from build123d import *

# Parameters (mm, degrees)
F1_DEPTH      = 125
F1_DEPTH_BACK = 125
F6_DEPTH      = 5.001
F7_DEPTH      = 30.001
F8_DEPTH      = 2
F9_DEPTH      = 2
F10_DEPTH     = 2
F11_DEPTH     = 2


with BuildPart() as f1:
    # F0 (on Front) → F1 (new body, two sides)
    with BuildSketch(Plane.XZ) as f1_sk:
        Polygon((15, -20), (15, 20), (-15, 20), (-15, -20), (-10, -20), (-10, 15), (10, 15), (10, -20), align=None)
    extrude(amount=F1_DEPTH)
    extrude(f1_sk.sketch, amount=-F1_DEPTH_BACK)

    # F4 (on face) → F6 (cut, through all)
    with BuildSketch(Plane.YZ.offset(-10)):
        with BuildLine():
            Line((107.5, 2.5), (-107.5, 2.5))
            ThreePointArc((-107.5, 2.5), (-112.5, -2.5), (-107.5, -7.5))
            Line((-107.5, -7.5), (107.5, -7.5))
            ThreePointArc((107.5, -7.5), (112.5, -2.5), (107.5, 2.5))
        make_face()
    extrude(amount=-F6_DEPTH, mode=Mode.SUBTRACT)

    # F2 (on face) → F7 (cut, through all)
    with BuildSketch(Plane(origin=(-15, 0, 0), x_dir=(0, -1, 0), z_dir=(-1, 0, 0))):
        with BuildLine():
            Line((-107.5, -7.5), (107.5, -7.5))
            ThreePointArc((107.5, -7.5), (112.5, -2.5), (107.5, 2.5))
            Line((107.5, 2.5), (-107.5, 2.5))
            ThreePointArc((-107.5, 2.5), (-112.5, -2.5), (-107.5, -7.5))
        make_face()
    extrude(amount=-F7_DEPTH, mode=Mode.SUBTRACT)

    # F5 (on face) → F8 (cut)
    with BuildSketch(Plane(origin=(10, 0, 0), x_dir=(0, -1, 0), z_dir=(-1, 0, 0))):
        with BuildLine():
            Line((107.5, 8.75), (-107.5, 8.75))
            ThreePointArc((-107.5, 8.75), (-118.75, -2.5), (-107.5, -13.75))
            Line((-107.5, -13.75), (107.5, -13.75))
            ThreePointArc((107.5, -13.75), (118.75, -2.5), (107.5, 8.75))
        make_face()
        with BuildLine():
            ThreePointArc((-107.5, -7.5), (-112.5, -2.5), (-107.5, 2.5))
            Line((-107.5, 2.5), (107.5, 2.5))
            ThreePointArc((107.5, 2.5), (112.5, -2.5), (107.5, -7.5))
            Line((107.5, -7.5), (-107.5, -7.5))
        make_face(mode=Mode.SUBTRACT)
    extrude(amount=-F8_DEPTH, mode=Mode.SUBTRACT)

    # F4 (on face) → F9 (cut)
    with BuildSketch(Plane.YZ.offset(-10)):
        with BuildLine():
            Line((107.5, 8.75), (-107.5, 8.75))
            ThreePointArc((-107.5, 8.75), (-118.75, -2.5), (-107.5, -13.75))
            Line((-107.5, -13.75), (107.5, -13.75))
            ThreePointArc((107.5, -13.75), (118.75, -2.5), (107.5, 8.75))
        make_face()
        with BuildLine():
            ThreePointArc((-107.5, -7.5), (-112.5, -2.5), (-107.5, 2.5))
            Line((-107.5, 2.5), (107.5, 2.5))
            ThreePointArc((107.5, 2.5), (112.5, -2.5), (107.5, -7.5))
            Line((107.5, -7.5), (-107.5, -7.5))
        make_face(mode=Mode.SUBTRACT)
    extrude(amount=-F9_DEPTH, mode=Mode.SUBTRACT)

    # F3 (on face) → F10 (cut)
    with BuildSketch(Plane.YZ.offset(15)):
        with BuildLine():
            ThreePointArc((-107.5, 8.75), (-118.75, -2.5), (-107.5, -13.75))
            Line((-107.5, -13.75), (107.5, -13.75))
            ThreePointArc((107.5, -13.75), (118.75, -2.5), (107.5, 8.75))
            Line((107.5, 8.75), (-107.5, 8.75))
        make_face()
        with BuildLine():
            ThreePointArc((-107.5, -7.5), (-112.5, -2.5), (-107.5, 2.5))
            Line((-107.5, 2.5), (107.5, 2.5))
            ThreePointArc((107.5, 2.5), (112.5, -2.5), (107.5, -7.5))
            Line((107.5, -7.5), (-107.5, -7.5))
        make_face(mode=Mode.SUBTRACT)
    extrude(amount=-F10_DEPTH, mode=Mode.SUBTRACT)

    # F2 (on face) → F11 (cut)
    with BuildSketch(Plane(origin=(-15, 0, 0), x_dir=(0, -1, 0), z_dir=(-1, 0, 0))):
        with BuildLine():
            Line((-107.5, -13.75), (107.5, -13.75))
            ThreePointArc((107.5, -13.75), (118.75, -2.5), (107.5, 8.75))
            Line((107.5, 8.75), (-107.5, 8.75))
            ThreePointArc((-107.5, 8.75), (-118.75, -2.5), (-107.5, -13.75))
        make_face()
        with BuildLine():
            ThreePointArc((107.5, 2.5), (112.5, -2.5), (107.5, -7.5))
            Line((107.5, -7.5), (-107.5, -7.5))
            ThreePointArc((-107.5, -7.5), (-112.5, -2.5), (-107.5, 2.5))
            Line((-107.5, 2.5), (107.5, 2.5))
        make_face(mode=Mode.SUBTRACT)
    extrude(amount=-F11_DEPTH, mode=Mode.SUBTRACT)


solid = f1.part
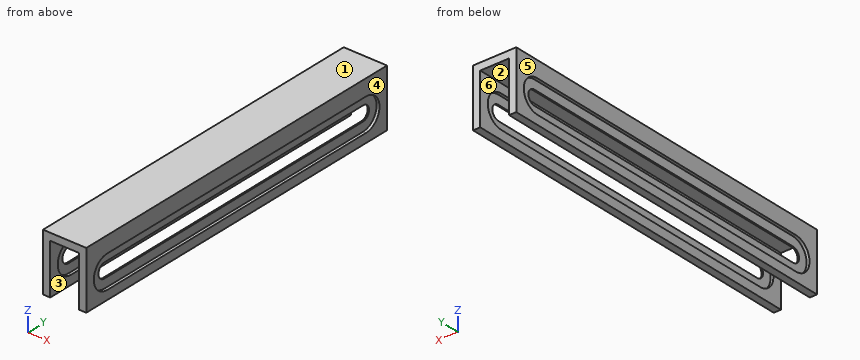
The model under review builds one solid part; all positions refer to its coordinate system, in mm. Face numbers are marked on the shaded views. A direction names the side the tool comes from. Coordinates: 2 decimals unless noted, no trailing zeros. Put each result on its own line as item: value.
1) Wall thickness on probe 1 along X at (y, z) = (-85, 11); probe 2 along Z at (x, y) = (11.5, 84); probe 3 along X at (y, z) = (-31, -9): over which ranges is each line inside the solid? List them lowest first. Write a range as [from, to].
Computed:
probe 1: x = [-15, -10], [10, 15]
probe 2: z = [-20, -13.75], [8.75, 20]
probe 3: x = [-13, -12], [12, 13]
2) Add section A-A on z = -2.5. State how many separate pieces and enclosed holes the cut face has, then the cut area to 3 significant figures.
Computed:
separate pieces: 4
enclosed holes: 0
area: 150 mm2
3) Draft analysis for pull direction X (two halves, no side actions). For the marked faces 1, 2, 3 and 4, state which applies: released by +X, released by -X, zero draft, split by the parting line, or undercut.
Computed:
face 1: zero draft
face 2: undercut
face 3: undercut
face 4: released by +X
4) Clearance check with flat-ended pins moving along their axes: pin 1 Ø5 at (y, z) = (-6, 6) entering from +X; pin 2 Ø8 at (x, y) = (0.5, -74) entering from -Z. State where each tip first meets the part, or that it passes through.
Computed:
pin 1: stops at x = 13
pin 2: stops at z = 15
5) For the marked faces 5 and 6, list the 3-axis set-ups (+Z, -Z, +X, -X, +Y, -Y) from which the entire face can be reached by the end or side of a thin tool; tool diameter is ignored.
Computed:
face 5: +Z, -Z, -X, +Y, -Y
face 6: -Z, +Y, -Y
